Input: part model. Units: mm. Frame: model coordinates. A direction names the side the tool comes from. Round coordinates to 2 decimals unless told otherwise and drop trailing zeros. Loops run counter-clockwise (first coordinate to the right, second up) from the corner with the lowest first, then second, coordinate; pieces in that order, holes last. Notation, with made-up numbers: M 58.25,0.25 L 110.25,0.25 A9 ccw 110.25,8.25 Z; hole C 89.5,19 d11. An arc over 180 degrees is marked long. Put each result on its own line as item: value. Start each with the question number.
1) Line query: probe 1 along Y at (x, z) = (0, 1.65); probe 2 along Y at (x, z) = (-13.5, 0.4); probe 3 along Y at (x, z) = (-37.5, 0.35). Output: solid intervals per line, ascending.
2) Section D-D on x = -90. Output: boundary loops of the cut face in (y, z), plus the area to 3 significant figures.
3) Draft query along Y for faces 3 (the face through (-27, 53, 3)), 4 (the face through (-24.93, 112.265, 1.479)), 5 (the face through (38.665, 39.116, 1.479)). Return one class per face: +Y half, -Y half, draft (parallel to the pull), parting line (faces both ways), or undercut.
4) Section A-A on z = 1.9. Output: boundary loops of the cut face in (x, y).
5) Pin query (flat end, axial travel): pin 1 (13.5 mm diameter, centred on x = -90, y = 0, fed in from +Z). Return the tip coordinate at first contact, or that it passes through.
6) Reachability of faces 1 (the face through (-38.665, -39.116, 1.479)), 2 (the face through (-27, 53, 0)) from +Z, -Z, +X, -X, +Y, -Y: full face, straight path, thin tool, end or side. Return the list, or none.
7) Section B-B on x = 0. Output: boundary loops of the cut face in (y, z).
Autodesk Inventor part; units mm, degrees
ref_plane "YZ Plane" through (0, 0, 0) normal (1, 0, 0) x (0, 1, 0)
ref_plane "XZ Plane" through (0, 0, 0) normal (0, 1, 0) x (-1, 0, 0)
ref_plane "XY Plane" through (0, 0, 0) normal (0, 0, 1) x (1, 0, 0)
sketch "Sketch1" plane through (0, 0, 0) normal (0, 0, 1) x (1, 0, 0)
  circle A0 centre (0, 0) radius 115
  line L0 (55, 55) -> (-55, 55)
  line L1 (-55, 55) -> (-55, -55)
  line L2 (-55, -55) -> (55, -55)
  line L3 (55, -55) -> (55, 55)
  line L4 (55, 55) -> (-55, -55) construction
  line L5 (-55, 55) -> (55, -55) construction
  line L6 (-55, 22.7817) -> (-22.7817, 55)
  line L7 (22.7817, 55) -> (55, 22.7817)
  line L8 (55, -22.7817) -> (22.7817, -55)
  line L9 (-22.7817, -55) -> (-55, -22.7817)
  dimension "d157" = 230
  dimension "d158" = 110
  dimension "d159" = 110
  dimension "d171" = 110
  dimension "d172" = 110
extrude "Plate5" add sketch "Sketch1" along normal blind 3 contours A0 | L3 L7 L0 | L6 L1 L0 | L3 L2 L8 | L9 L2 L1
sketch "Sketch7" plane through (0, 0, 0) normal (0, 0, -1) x (-1, 0, 0)
  circle A0 centre (0, 90) radius 8.5
  circle A1 centre (0, 0) radius 90 construction
  dimension "d170" = 180
  dimension "d160" = 17
extrude "Cut1" cut sketch "Sketch7" against normal blind 3
pattern_circular "Circular Pattern1" count 4 over 360 about axis through (0, 0, -10) along (0, 0, 1) of "Cut1"
properties part number "APN 1472  funnel FLANGE 1200 50-90" material "Stainless Steel"
Geometry results:
1. probe 1: y = -115 to -98.5, -81.5 to -55, 55 to 81.5, 98.5 to 115
1. probe 2: y = -114.2 to -55, 55 to 114.2
1. probe 3: y = -108.71 to -40.28, 40.28 to 108.71
2. outline: M -71.59,0 L -8.5,0 L -8.5,3 L -71.59,3 Z; M 8.5,0 L 71.59,0 L 71.59,3 L 8.5,3 Z
2. area: 379 mm²
3. face 3: draft
3. face 4: parting line
3. face 5: undercut
4. outline: C 0,0 d230; hole C -90,0 d17; hole M -55,-22.78 L -22.78,-55 L 22.78,-55 L 55,-22.78 L 55,22.78 L 22.78,55 L -22.78,55 L -55,22.78 Z; hole C 0,-90 d17; hole C 0,90 d17; hole C 90,0 d17
5. pin 1: passes through
6. face 1: +Z, -Z
6. face 2: -Z, +X, -X, +Y, -Y
7. outline: M -115,0 L -98.5,0 L -98.5,3 L -115,3 Z; M -81.5,0 L -55,0 L -55,3 L -81.5,3 Z; M 55,0 L 81.5,0 L 81.5,3 L 55,3 Z; M 98.5,0 L 115,0 L 115,3 L 98.5,3 Z
